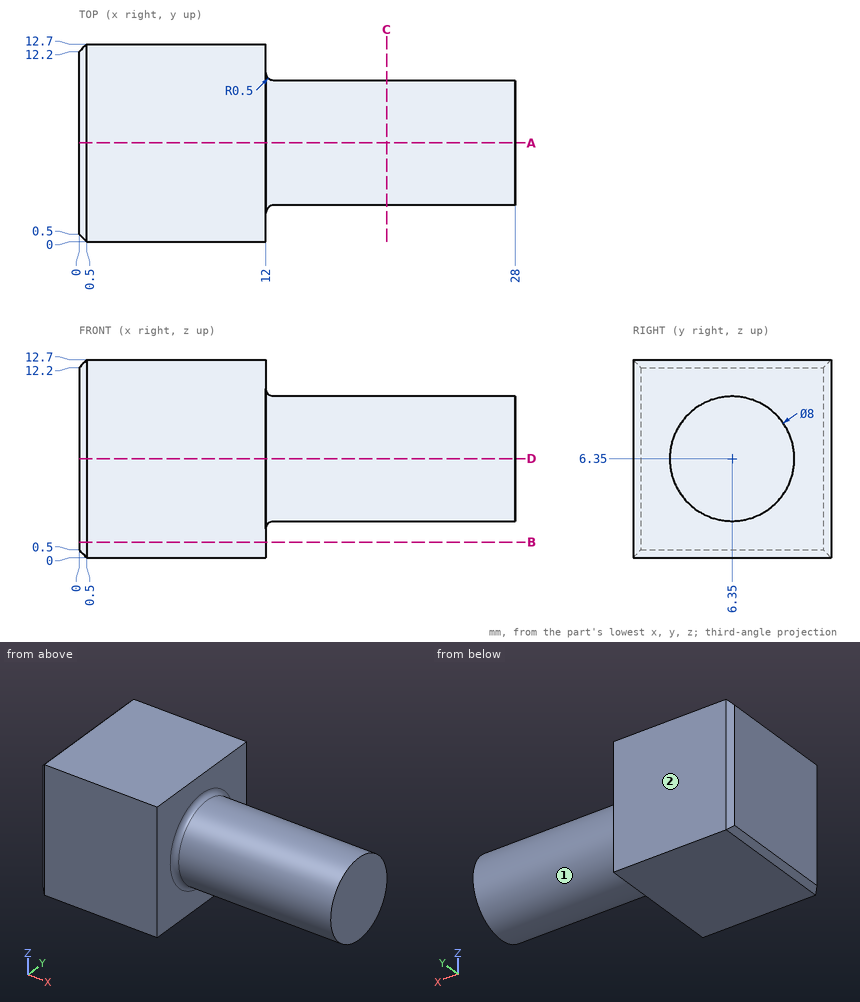
The figure shows three views and two pictorial views of one solid part (mm, origin at its lowest corner). Answer the questions. A direction names the side the tool comes from. Give positions to 0.01 mm unless a question says otherwise; leave off trailing zeros. Write each loop counter-clockwise with the first axis right and the second up, starting at its lowest first coordinate (ties: lowest second). Pieces come first, ordered by that corner, then holes. Notation, with made-up numbers: (-17, 28) - (24, 28) arc R22 cw to (24, 52) - close; hole circle Ø10 at (0, -3). An arc over 180 degrees is marked (long way). Return JSON: item names as keys, results as strings.
Q1. For the marked faces 1 and 2, determine the directions among +Z, -Z, +X, -X, +Y, -Y from which every point of the face is accessible in a straight line to the end or side of a thin tool.
Reply:
{"face 1": "+X", "face 2": "+Z, -Z, +X, -X, +Y"}
Q2. Consider line 1 along X through (y, z) = (9, 11.5); line 2 along Y through (x, z) = (14.25, 6); line 3 along Z through (x, y) = (26.5, 7.75). Determine where each line is inside the solid, lowest interval first. Write a range as [from, to].
Reply:
{"line 1": "[0, 12]", "line 2": "[2.37, 10.33]", "line 3": "[2.6, 10.1]"}
Q3. Given P1, Ø2, axis at x = 17.5, z = 3, coming from the +Y side; P2, Ø3, axis at x = 22, y = 3, coming from the +Z side; P3, Ø5, axis at x = 19, y = 8.5, coming from the -Z side, each flat-ended and moving along its own axis, determine where each tip first touches the part or whether it passes through.
Reply:
{"P1": "y = 9.59", "P2": "z = 9.9", "P3": "z = 2.35"}
Q4. A cutting plane is placed at A-A, the plane y = 6.35. Determine the outline of the cut face in (x, z), and give its area (3 significant figures).
Reply:
{"outline": "(0, 0.5) - (0.5, 0) - (12, 0) - (12, 1.85) arc R0.5 cw to (12.5, 2.35) - (28, 2.35) - (28, 10.35) - (12.5, 10.35) arc R0.5 cw to (12, 10.85) - (12, 12.7) - (0.5, 12.7) - (0, 12.2) - close", "area": "280 mm²"}
Q5. A cutting plane is placed at B-B, the plane z = 1. Determine the outline of the cut face in (x, y).
Reply:
{"outline": "(0, 0.5) - (0.5, 0) - (12, 0) - (12, 12.7) - (0.5, 12.7) - (0, 12.2) - close"}
Q6. A cutting plane is placed at C-C, the plane x = 19.75. Determine the outline of the cut face in (y, z), and give its area (3 significant figures).
Reply:
{"outline": "circle Ø8 at (6.35, 6.35)", "area": "50.3 mm²"}
